```python
from build123d import *

# Parameters (mm, degrees)
SKETCH2_W           = 3.81
SKETCH2_H           = 25.4
BOSS_EXTRUDE1_DEPTH = 5.334
SKETCH3_OUTSIDE_W   = 11.056
SKETCH3_OUTSIDE_H   = 32.646
CUT_EXTRUDE1_DEPTH  = 27.232187404


with BuildPart() as part:
    # Sketch2 → Boss-Extrude1 (new body)
    with BuildSketch(Plane(origin=(0, 0, 0), x_dir=(1, 0, 0), z_dir=(0, 1, 0))):
        with Locations((1.905, 12.7)):
            Rectangle(SKETCH2_W, SKETCH2_H)
    extrude(amount=BOSS_EXTRUDE1_DEPTH)

    # Sketch3 outside → Cut-Extrude1 (cut, through all)
    with BuildSketch(Plane(origin=(0, 5.334, 0), x_dir=(1, 0, 0), z_dir=(0, 1, 0))):
        with Locations((1.905, 12.7)):
            Rectangle(SKETCH3_OUTSIDE_W, SKETCH3_OUTSIDE_H)
        Polygon((0.762, 5.08), (2.61096879, 0), (3.81, 0), (3.81, 25.4), (0, 25.4), (0, 6.858), (2.286, 6.858), (2.286, 5.08), align=None, mode=Mode.SUBTRACT)
    extrude(amount=-CUT_EXTRUDE1_DEPTH, mode=Mode.SUBTRACT)


solid = part.part
```
Check sheet for the modelled part. Datum: model origin and axes. Units: mm. A direction names the side the tool comes from. Give positions to 0.01 mm unless a question says otherwise; leave off trailing zeros. Write each loop counter-clockwise with the first axis right and the second up, starting at its lowest first coordinate (ties: lowest second). Pieces come first, ordered by that corner, then holes.
Item 1: Cross-section at C-C (z = -4). Enter the section's corners in (x, y), and give its area (3 significant figures).
Item 2: Access from +Z, -Z, +X, -X, +Y, -Y to the whole of each face (thin tool, end or side, straight path). Record for faces 1 (the face through (2, 3, -5.08)), 2 (the face through (3, 3, 0)).
Item 3: Scan lines: L1, parallel to Z at x = 0.7, y = 4.15; L2, parallel to X at y = 4.65, z = -2.5; L3, parallel to X at y = 2, z = -3.5. Record each from-to range of solid material in increasing order.
Item 4: Gauge pin test, flat end, axial feed: pin 1 (1.4 mm diameter, centred on y = 3.5, z = -6, fed in from -X). Record the tip position at first contact, or that the pin passes through.
Item 5: Cross-section at A-A (x = 1.8). Enter the section's corners in (y, z).
Item 6: Cross-section at B-B (y = 0.8). Enter the section's corners in (x, z).
Item 7: Draft check along Z on faces 3 (the face through (3.81, 3, -13)), 4 (the face through (1.67, 2.7, -2.58)), 5 (the face through (1, 3, -6.858)). Enter one of: released by +Z, released by -Z, zero draft, split by the parting line, or undercut.
Report:
1. outline: (1.16, 0) - (3.81, 0) - (3.81, 5.33) - (1.16, 5.33) - close
1. area: 14.2 mm2
2. face 1: -X, +Y, -Y
2. face 2: +Z, +X, -X, +Y, -Y
3. L1: z = -25.4 to -6.86
3. L2: x = 1.7 to 3.81
3. L3: x = 1.34 to 3.81
4. pin 1: stops at x = 2.29
5. outline: (0, -25.4) - (5.33, -25.4) - (5.33, -6.86) - (0, -6.86) - close; (0, -5.08) - (5.33, -5.08) - (5.33, -2.23) - (0, -2.23) - close
6. outline: (0, -25.4) - (3.81, -25.4) - (3.81, 0) - (2.61, 0) - (0.76, -5.08) - (2.29, -5.08) - (2.29, -6.86) - (0, -6.86) - close
7. face 3: zero draft
7. face 4: released by +Z
7. face 5: undercut
